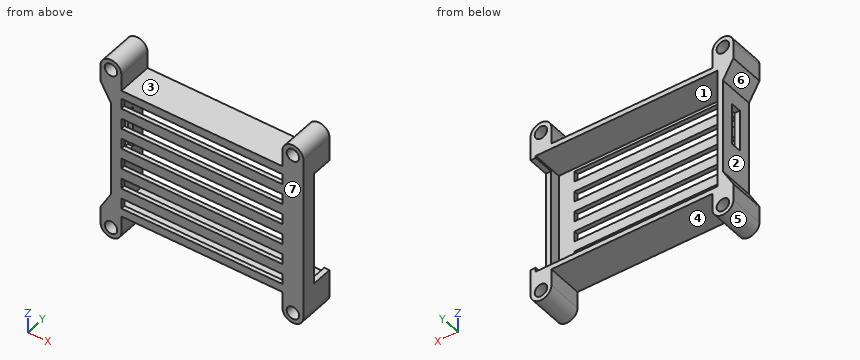
```python
from build123d import *

# Parameters (mm, degrees)
BOSS_EXTRUDE1_DEPTH = 2
SKETCH6_W           = 87
SKETCH6_H           = 58.002207555
BOSS_EXTRUDE3_DEPTH = 15
SKETCH10_W          = 2.5
SKETCH10_H          = 55.002207555
CUT_EXTRUDE2_DEPTH  = 10
HOLE5_START         = -1
HOLE5_OUTLINE_R     = 3
HOLE5_DEPTH         = 18
SKETCH15_W          = 20
SKETCH15_H          = 5
CUT_EXTRUDE4_DEPTH  = 2.5
SKETCH_2_W          = 77
SKETCH_2_H          = 5
SKETCH_2_H_2        = 5.00441511
CUT_EXTRUDE_4_DEPTH = 10


with BuildPart() as part:
    # Sketch1 → Boss-Extrude1 (new body)
    with BuildSketch(Plane(origin=(0, 0, 0), x_dir=(1, 0, 0), z_dir=(0, 1, 0))):
        with BuildLine():
            Line((-46, 22.841953517), (-46, -22.841953517))
            Line((-46, -22.841953517), (-51, -31.502207555))
            Line((-51, -31.502207555), (-51, -39.502207555))
            ThreePointArc((-51, -39.502207555), (-46, -44.502207555), (-41, -39.502207555))
            Line((-41, -39.502207555), (-41, -31.502207555))
            Line((-41, -31.502207555), (36, -31.502207555))
            Line((36, -31.502207555), (36, -39.502207555))
            ThreePointArc((36, -39.502207555), (41, -44.502207555), (46, -39.502207555))
            Line((46, -39.502207555), (46, 39.502207555))
            ThreePointArc((46, 39.502207555), (41, 44.502207555), (36, 39.502207555))
            Line((36, 39.502207555), (36, 31.502207555))
            Line((36, 31.502207555), (-41, 31.502207555))
            Line((-41, 31.502207555), (-41, 39.502207555))
            ThreePointArc((-41, 39.502207555), (-46, 44.502207555), (-51, 39.502207555))
            Line((-51, 39.502207555), (-51, 31.502207555))
            Line((-51, 31.502207555), (-46, 22.841953517))
        make_face()
    extrude(amount=BOSS_EXTRUDE1_DEPTH)

    # Sketch6 → Boss-Extrude3 (add)
    with BuildSketch(Plane(origin=(0, 2, 0), x_dir=(1, 0, 0), z_dir=(0, 1, 0))):
        with BuildLine():
            Line((-46, -22.841953517), (-51, -31.502207555))
            Line((-51, -31.502207555), (-51, -39.502207555))
            ThreePointArc((-51, -39.502207555), (-46, -44.502207555), (-41, -39.502207555))
            Line((-41, -39.502207555), (-41, -31.502207555))
            Line((-41, -31.502207555), (36, -31.502207555))
            Line((36, -31.502207555), (36, -39.502207555))
            ThreePointArc((36, -39.502207555), (41, -44.502207555), (46, -39.502207555))
            Line((46, -39.502207555), (46, 39.502207555))
            ThreePointArc((46, 39.502207555), (41, 44.502207555), (36, 39.502207555))
            Line((36, 39.502207555), (36, 31.502207555))
            Line((36, 31.502207555), (-41, 31.502207555))
            Line((-41, 31.502207555), (-41, 39.502207555))
            ThreePointArc((-41, 39.502207555), (-46, 44.502207555), (-51, 39.502207555))
            Line((-51, 39.502207555), (-51, 31.502207555))
            Line((-51, 31.502207555), (-46, 22.841953517))
            Line((-46, 22.841953517), (-46, -22.841953517))
        make_face()
        with Locations((0, -0.001103777)):
            Rectangle(SKETCH6_W, SKETCH6_H, mode=Mode.SUBTRACT)
    extrude(amount=BOSS_EXTRUDE3_DEPTH)

    # Sketch10 → Cut-Extrude2 (cut)
    with BuildSketch(Plane(origin=(0, 17, 0), x_dir=(1, 0, 0), z_dir=(0, 1, 0))):
        with Locations((44.75, -0.501103778)):
            Rectangle(SKETCH10_W, SKETCH10_H)
    extrude(amount=-CUT_EXTRUDE2_DEPTH, mode=Mode.SUBTRACT)

    # Hole5: read off the stored shape, not the designer's step
    # Hole5 outline → Hole5 (cut)
    with BuildSketch(Plane(origin=(0, 0, 0), x_dir=(1, 0, 0), z_dir=(0, 1, 0)).offset(HOLE5_START)):
        with Locations((-46, -39.502207555)):
            Circle(HOLE5_OUTLINE_R)
        with Locations((41, -39.502207555)):
            Circle(HOLE5_OUTLINE_R)
        with Locations((41, 39.502207555)):
            Circle(HOLE5_OUTLINE_R)
        with Locations((-46, 39.502207555)):
            Circle(HOLE5_OUTLINE_R)
    extrude(amount=HOLE5_DEPTH, mode=Mode.SUBTRACT)

    # Sketch15 → Cut-Extrude4 (cut)
    with BuildSketch(Plane.ZY.offset(46)):
        with Locations((5, 8.5)):
            Rectangle(SKETCH15_W, SKETCH15_H)
    extrude(amount=-CUT_EXTRUDE4_DEPTH, mode=Mode.SUBTRACT)

    # 草图2 → 切除-拉伸4 (cut)
    with BuildSketch(Plane.XZ):
        with Locations((-2.5, -25.002207555)):
            Rectangle(SKETCH_2_W, SKETCH_2_H)
        with Locations((-2.5, -15.002207555)):
            Rectangle(SKETCH_2_W, SKETCH_2_H)
        with Locations((-2.5, -5.002207555)):
            Rectangle(SKETCH_2_W, SKETCH_2_H)
        with Locations((-2.5, 4.997792445)):
            Rectangle(SKETCH_2_W, SKETCH_2_H)
        with Locations((-2.5, 14.997792445)):
            Rectangle(SKETCH_2_W, SKETCH_2_H)
        with Locations((-2.5, 25)):
            Rectangle(SKETCH_2_W, SKETCH_2_H_2)
    extrude(amount=-CUT_EXTRUDE_4_DEPTH, mode=Mode.SUBTRACT)


solid = part.part
```
Could you check a few things on this model? Use its own coordinates, in mm. Face numbers are marked on the shaded views. A direction names the side the tool comes from. Give positions to 0.01 mm unless a question says otherwise; leave off trailing zeros. Write each loop counter-clockwise with the first axis right and the second up, starting at its lowest first coordinate (ties: lowest second). Pieces come first, ordered by that corner, then holes. Notation, with made-up numbers: (34, 78) -> (60, 78) arc R20 ccw to (60, 111) -> close; hole circle Ø1 at (33, -8). An arc over 180 degrees is marked (long way). Write each question's results on one line, items separated by ' | '.
1. On a 3-axis mill with a long thin cutter (end or side, diameter ignored), from which of +Z, -Z, +X, -X, +Y, -Y can I reach the whole of each face in a straight line? I mean the marked faces 1, 2, 3 and 4. Say none if no direction works.
Check sheet entries:
face 1: +Y | face 2: -X, +Y, -Y | face 3: +Z, +Y, -Y | face 4: -Z, +Y, -Y
2. I want a section at D-D, the plane y = 15.5. Write out the boundary of the cut face in (x, z).
Check sheet entries:
outline: (-51, -39.5) arc R5 ccw to (-41, -39.5) -> (-41, -31.5) -> (36, -31.5) -> (36, -39.5) arc R5 ccw to (46, -39.5) -> (46, -27) -> (43.5, -27) -> (43.5, -29) -> (-43.5, -29) -> (-43.5, 29) -> (43.5, 29) -> (43.5, 28) -> (46, 28) -> (46, 39.5) arc R5 ccw to (36, 39.5) -> (36, 31.5) -> (-41, 31.5) -> (-41, 39.5) arc R5 ccw to (-51, 39.5) -> (-51, 31.5) -> (-46, 22.84) -> (-46, -22.84) -> (-51, -31.5) -> close; hole circle Ø6 at (-46, -39.5); hole circle Ø6 at (-46, 39.5); hole circle Ø6 at (41, -39.5); hole circle Ø6 at (41, 39.5)
3. I need wall thicknesses on L1, parallel to Z at x = 41, y = 10.75; L2, parallel to Z at x = -4, y = 2.75; L3, parallel to X at y = 3, z = 20.5. Which ranges of each line are inside material? Lowest first, please.
Check sheet entries:
L1: z = -44.5 to -42.5, -36.5 to -29, 29 to 36.5, 42.5 to 44.5 | L2: z = -31.5 to -29, 29 to 31.5 | L3: x = -46 to -43.5, 43.5 to 46
4. If we mould it in two halves opening along Z, with no side actions, what happens to the marked faces 5, 6 and 7? For each: released by +Z, released by -Z, zero draft, split by the parting line, or undercut.
Check sheet entries:
face 5: released by -Z | face 6: undercut | face 7: zero draft
5. I want a section at A-A, the plane y = 8.5. Count the separate pieces of the cut face and the enclosed holes in it, then the cut area to 3 significant figures.
Check sheet entries:
separate pieces: 2 | enclosed holes: 4 | area: 970 mm²
6. I want a section at B-B, the plane x = 41. Write out the boundary of the cut face in (y, z), then the cut area to 3 significant figures.
Check sheet entries:
outline: (0, -44.5) -> (17, -44.5) -> (17, -42.5) -> (0, -42.5) -> close; (0, -36.5) -> (17, -36.5) -> (17, -29) -> (2, -29) -> (2, 29) -> (17, 29) -> (17, 36.5) -> (0, 36.5) -> close; (0, 42.5) -> (17, 42.5) -> (17, 44.5) -> (0, 44.5) -> close | area: 439 mm²
7. Will these pins go through, and if not, where does the flat tip stop? pin 1 Ø0.6 at (x, y) = (-17.5, 1.5) entering from +Z; pin 2 Ø1.2 at (x, y) = (45, 13.5) entering from -Z; pin 3 Ø12 at (x, z) = (34, -17) entering from +Y; pin 4 Ø5.5 at (x, z) = (41, -39.5) entering from +Y.
Check sheet entries:
pin 1: stops at z = 31.5 | pin 2: stops at z = -43.17 | pin 3: stops at y = 2 | pin 4: passes through
8. I want a section at C-C, the plane z = 5.5. Write out the boundary of the cut face in (x, y).
Check sheet entries:
outline: (-46, 0) -> (-41, 0) -> (-41, 2) -> (-43.5, 2) -> (-43.5, 6) -> (-46, 6) -> close; (-46, 11) -> (-43.5, 11) -> (-43.5, 17) -> (-46, 17) -> close; (36, 0) -> (46, 0) -> (46, 7) -> (43.5, 7) -> (43.5, 2) -> (36, 2) -> close
